from build123d import *


with BuildPart() as part:
    # Sketch1 → Revolve1 (revolve)
    with BuildSketch(Plane(origin=(0, 0, 0), x_dir=(-1, 0, 0), z_dir=(0, 0, -1))):
        with BuildLine():
            Line((-1, 11), (-1, 3))
            add(Edge.make_bspline(
                [(-1, 3), (-1.078203591, 2.575668755), (-1.2, 2.5)],
                knots=[0, 0, 0, 0.432994338, 0.432994338, 0.432994338], degree=2))
            add(Edge.make_bspline(
                [(-1, 2), (-1.078203591, 2.424331245), (-1.2, 2.5)],
                knots=[0, 0, 0, 0.432994338, 0.432994338, 0.432994338], degree=2))
            Line((-1, 2), (0, 2))
            Line((0, 2), (0, 12.25))
            ThreePointArc((0, 12.25), (-0.073223305, 12.426776695), (-0.25, 12.5))
            Line((-0.25, 12.5), (-1, 12.5))
            ThreePointArc((-1, 12.5), (-1.75, 11.75), (-1, 11))
        make_face()
    revolve(axis=Axis((-1.443304251, 0, 0), (1, 0, 0)))


solid = part.part
The listing builds one solid part. Answer for the finished solid, in the listing's coordinates (mm). Coordinates: 2 decimals unless noted, no trailing zeros. One line per question, with ' | ' between items.
1. Given pin 1 Ø3 at (y, z) = (9.5, -10) entering from -X; pin 2 Ø1 at (x, z) = (1, -4.5) entering from -Y, each flat-ended and moving along its own axis, determine where each tip first touches the part or whether it passes through.
Verdict:
pin 1: stops at x = 0 | pin 2: stops at y = -11.84
2. For a pull along Z with two mould halves and no side action, classify faces 1 (the flat face through (1, 2.3, -2.3)), 2 (the flat face through (0, -3, 0)), 3 (the cylindrical face through (0.63, 11.923, 3.755)) as released by +Z, released by -Z, zero draft, split by the parting line, or undercut.
Verdict:
face 1: undercut | face 2: zero draft | face 3: split by the parting line
3. Straight lines are drawn through the part: line 1 (Z direction, x = 0.45, y = 0); line 2 (X direction, y = -10.5, z = -2.5); line 3 (Z direction, x = 1.25, y = 7.75). For each, find the intervals that lie inside material, in ascending order.
Verdict:
line 1: z = -12.5 to -2, 2 to 12.5 | line 2: x = 0 to 1 | line 3: z = -9.75 to -7.87, 7.87 to 9.75
